The listing builds one solid part. Answer for the finished solid, in the listing's coordinates (mm). Face numbers are marked on the shaded views. A direction names the side the tool comes from. Give positions to 0.01 mm unless a question says otherwise; leave off trailing zeros. Write each loop counter-clockwise with the first axis right and the second up, starting at its lowest first coordinate (ties: lowest second). Pieces come first, ordered by that corner, then holes.
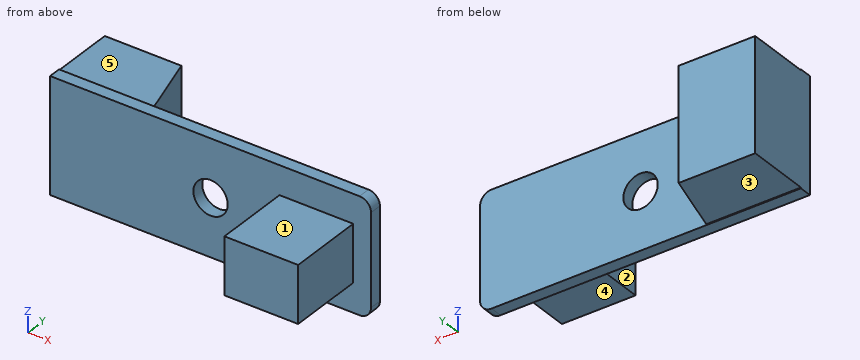
```python
from build123d import *

# Parameters (mm, degrees)
SKETCH1_R           = 1.5
BOSS_EXTRUDE1_DEPTH = 1.08
SKETCH2_W           = 6.68
SKETCH2_H           = 9.85
BOSS_EXTRUDE2_DEPTH = 5.54
BOSS_EXTRUDE3_DEPTH = 9.85
SKETCH4_W           = 6.43
SKETCH4_H           = 4.96
BOSS_EXTRUDE4_DEPTH = 6.67


with BuildPart() as part:
    # Sketch1 → Boss-Extrude1 (new body)
    with BuildSketch(Plane(origin=(0, 0, 0), x_dir=(1, 0, 0), z_dir=(0, 1, 0))):
        with BuildLine():
            Line((0, 0), (27, 0))
            ThreePointArc((27, 0), (27.707106781, 0.292893219), (28, 1))
            Line((28, 1), (28, 9))
            ThreePointArc((28, 9), (27.707106781, 9.707106781), (27, 10))
            Line((27, 10), (0, 10))
            Line((0, 10), (0, 0))
        make_face()
        with Locations(Location((14, 5, 0), (0, 0, 270))):
            Circle(SKETCH1_R, mode=Mode.SUBTRACT)
    extrude(amount=BOSS_EXTRUDE1_DEPTH)

    # Sketch2 → Boss-Extrude2 (add)
    with BuildSketch(Plane(origin=(0, 1.08, 0), x_dir=(1, 0, 0), z_dir=(0, 1, 0))):
        with Locations((3.34, 5)):
            Rectangle(SKETCH2_W, SKETCH2_H)
    extrude(amount=BOSS_EXTRUDE2_DEPTH)

    # Sketch3 → Boss-Extrude3 (add)
    with BuildSketch(Plane.XY.offset(-0.075)):
        Polygon((0, 1.08), (8.264602566, 1.08), (6.68, 6.62), (0, 6.62), align=None)
    extrude(amount=-BOSS_EXTRUDE3_DEPTH)

    # Sketch4 → Boss-Extrude4 (add)
    with BuildSketch(Plane.XZ):
        with Locations((23.235, -5)):
            Rectangle(SKETCH4_W, SKETCH4_H)
    extrude(amount=BOSS_EXTRUDE4_DEPTH)


solid = part.part
```
Item 1: A cutting plane is placed at C-C, the plane x = 26. Give the vertices of the cut face in (y, z).
Conclusion:
outline: (-6.67, -7.48) - (0, -7.48) - (0, -10) - (1.08, -10) - (1.08, 0) - (0, 0) - (0, -2.52) - (-6.67, -2.52) - close
Item 2: Each of these flat-tipped pins is pushed along its axis until it touches: P1, Ø3.5, axis at x = 14, z = -5, coming from the -Y side; P2, Ø2.5, axis at y = -2.5, z = -4, coming from the -X side; P3, Ø1.5, axis at y = -3.5, z = -4, coming from the +X side; P4, Ø1.5, axis at x = 12, y = 3.5, coming from the -Z side (3 decimals). Where does it stop, or does it pass through?
Conclusion:
P1: stops at y = 0
P2: stops at x = 20.02
P3: stops at x = 26.45
P4: passes through
Item 3: Which of the six approach directions +Z, -Z, +X, -X, +Y, -Y give full straight-line access (tool end or side, diameter ignored) to the marked faces 1, 2, 3, 4 and 5?
Conclusion:
face 1: +Z, +X, -X, -Y
face 2: +Z, -Z, -X, -Y
face 3: -Z, +X, -X, +Y
face 4: -Z, +X, -X, -Y
face 5: +Z, +X, -X, +Y
Item 4: A cutting plane is placed at B-B, the plane z = -5. Give the vertices of the cut face in (x, y), plus the area to 3 significant figures.
Conclusion:
outline: (0, 0) - (12.5, 0) - (12.5, 1.08) - (8.26, 1.08) - (6.68, 6.62) - (0, 6.62) - close; (15.5, 0) - (20.02, 0) - (20.02, -6.67) - (26.45, -6.67) - (26.45, 0) - (28, 0) - (28, 1.08) - (15.5, 1.08) - close
area: 111 mm2
Item 5: A cutting plane is placed at A-A, the plane x = 14. Give the vertices of the cut face in (y, z).
Conclusion:
outline: (0, -10) - (1.08, -10) - (1.08, -6.5) - (0, -6.5) - close; (0, -3.5) - (1.08, -3.5) - (1.08, 0) - (0, 0) - close
Item 6: A cutting plane is placed at D-D, the plane z = -2.25. Give the vertices of the cut face in (x, y), plus the area to 3 significant figures.
Conclusion:
outline: (0, 0) - (28, 0) - (28, 1.08) - (8.26, 1.08) - (6.68, 6.62) - (0, 6.62) - close
area: 71.6 mm2
Item 7: Consider probe 1 along X at (y, z) = (0.3, -5); probe 2 along Y at (x, z) = (22.5, -2.25); probe 3 along X at (y, z) = (-3.75, -4.75). Determine where each line is inside the solid, lowest interval first.
Conclusion:
probe 1: x = 0 to 12.5, 15.5 to 28
probe 2: y = 0 to 1.08
probe 3: x = 20.02 to 26.45
